Autodesk Inventor part; units mm, degrees
ref_plane "YZ Plane" through (0, 0, 0) normal (1, 0, 0) x (0, 1, 0)
ref_plane "XZ Plane" through (0, 0, 0) normal (0, 1, 0) x (-1, 0, 0)
ref_plane "XY Plane" through (0, 0, 0) normal (0, 0, 1) x (1, 0, 0)
sketch "Sketch1" plane through (0, 0, 0) normal (0, 1, 0) x (-1, 0, 0)
  line L0 (0, 0) -> (29.6, 0)
  line L1 (29.6, 0) -> (29.6, 24.2)
  line L2 (29.6, 24.2) -> (0, 24.2)
  line L3 (0, 24.2) -> (0, 0)
  line L4 (29.6, 12.5) -> (0, 12.5)
  line L5 (0, 12.5) -> (0, 0)
  line L6 (0, 0) -> (29.6, 0)
  line L7 (29.6, 0) -> (29.6, 12.5)
  line L8 (23.8, 24.2) -> (10.8, 24.2)
  line L9 (10.8, 24.2) -> (10.8, 12.5)
  line L10 (10.8, 12.5) -> (23.8, 12.5)
  line L11 (23.8, 12.5) -> (23.8, 24.2)
  line L12 (23.8, 17.7) -> (17.8, 17.7)
  line L13 (17.8, 17.7) -> (17.8, 12.5)
  line L14 (17.8, 12.5) -> (23.8, 12.5)
  line L15 (23.8, 12.5) -> (23.8, 17.7)
  line L16 (17.8, 17.7) -> (10.8, 17.7)
  line L17 (10.8, 17.7) -> (10.8, 12.5)
  line L18 (10.8, 12.5) -> (17.8, 12.5)
  line L19 (17.8, 12.5) -> (17.8, 17.7)
  circle A0 centre (21.6, 8) radius 8
  circle A1 centre (5, 7.5) radius 5
  circle A2 centre (16.3, 14) radius 1.5
  circle A3 centre (16.3, 16.2) radius 1.5
  circle A4 centre (26.8, 15.5) radius 3
  circle A5 centre (22.3, 22.7) radius 1.5
  circle A6 centre (11.8, 18.7) radius 1
  line L20 (10.8, 24.2) -> (15.8, 24.2)
  line L21 (15.8, 24.2) -> (15.8, 20.95)
  line L22 (15.8, 20.95) -> (10.8, 20.95)
  line L23 (10.8, 20.95) -> (10.8, 24.2)
  arc A7 (15.8, 24.2) -> (10.8, 20.95) centre (17.6697, 15.8525) ccw
  circle A8 centre (28.1, 11) radius 1.5
  point P0 (17.8, 14)
  point P1 (16.3, 12.5)
  point P2 (5, 12.5)
  point P3 (0, 7.5)
  point P4 (21.6, 0)
  point P5 (29.6, 8)
  point P6 (26.8, 12.5)
  point P7 (23.8, 15.5)
  point P8 (23.8, 22.7)
  point P9 (22.3, 24.2)
  point P10 (10.8, 18.7)
  point P11 (11.8, 17.7)
  point P12 (16.3, 17.7)
  point P13 (17.8, 16.2)
  point P14 (29.6, 11)
  point P15 (28.1, 12.5)
  dimension "d0" = 24.2
  dimension "d1" = 29.6
  dimension "d2" = 11.7
  dimension "d3" = 5.8
  dimension "d4" = 13
  dimension "d5" = 6.5
  dimension "d6" = 6
  dimension "d7" = 16
  dimension "d8" = 8
  dimension "d9" = 8
  dimension "d10" = 10
  dimension "d11" = 5
  dimension "d12" = 5
  dimension "d13" = 3
  dimension "d14" = 3
  dimension "d15" = 1.5
  dimension "d16" = 1.5
  dimension "d17" = 1.5
  dimension "d18" = 1.5
  dimension "d19" = 6
  dimension "d20" = 3
  dimension "d21" = 3
  dimension "d23" = 1.5
  dimension "d24" = 1.5
  dimension "d25" = 2
  dimension "d26" = 1
  dimension "d27" = 1
  dimension "d28" = 5
  dimension "d29" = 3.25
  dimension "d32" = 3
  dimension "d33" = 1.5
  dimension "d34" = 1.5
  dimension "d35" = 12.5
  dimension "d36" = 3
extrude "Extrusion1" add sketch "Sketch1" along normal blind 3 contours L3 A1 L4 A0 L0 | A0 L4 A8 | A1 | A0 A8 L1 | A2 L13 L4 | A8 A0 | A8 A0 | L13 A0 L11 L4 | L11 A4 L4 | L13 L12 L11 A0 | L9 L22 L21 L2 A5 L11 L12 L16 A6 | A6 | L16 L13 A3 | L21 L22 A7 | A5 picked at (19.8309, 8.6369)
properties part number "Pi_mount_newupper"
Could you check a few things on this model? Use its own coordinates, in mm. A direction names the side the tool comes from. Round coordinates to 2 decimals unless told otherwise and drop trailing zeros. Write each loop counter-clockwise with the first axis right and the second up, starting at its lowest first coordinate (ties: lowest second). Pieces come first, ordered by that corner, then holes. Notation, with made-up numbers: (-6, 26.25) - (3, 26.25) arc R4 cw to (3, 30.25) - close; hole circle Ø10 at (62, 79). An arc over 180 degrees is marked (long way). Put each result on its own line as item: value. Start each with the question number.
(1) For faces 1 (the flat face through (-10.8, 1, 20)), 2 (the cylindrical face through (-27.319, 1.479, 2.406)), 3 (the flat face through (-27, 1, 12.5)), 4 (the cylindrical face through (-17.35, 1.48, 17.27)), which set-ups out of +Z, -Z, +X, -X, +Y, -Y let a thin tool reach every point of the face, with its end or its side?
(2) I want a section at A-A, the plane x = -11.25. Please give me the cut outline in (y, z).
(3) Thinking about a two-plate mould opening in Z: for faces 5 (the flat face through (-15, 0, 10)), 6 (the flat face through (-17.8, 1, 15)), 7 (the flat face through (-11, 1, 0)), which applies, released by +Z, released by -Z, zero draft, split by the parting line, or undercut?
(4) I want a section at C-C, the plane z = 10.5. Please give me the cut outline in (x, y).
(5) Will these pins go through, and if not, where does the flat tip stop? pin 1 (1.1 mm diameter, centred on y = 1.5, z = 14.5, fed in from +X); pin 2 (5 mm diameter, centred on x = -10, z = 12.5, fed in from -Y); pin 3 (1 mm diameter, centred on x = -27, y = 2, fed in from +Z); pin 4 (1.5 mm diameter, centred on y = 0.5, z = 5.5, fed in from -X).
(6) I need wall thicknesses on probe 1 along Z at (x, y) = (-9.25, 2.2); probe 2 along X at (y, z) = (2, 15.5); probe 3 along X at (y, z) = (1.6, 18.75). Which ranges of each line are inside material? Lowest first, please.
(7) I want a section at B-B, the plane y = 0.5. Please give me the cut outline in (x, z), plus the area to 3 significant figures.
(8) I want a section at D-D, the plane z = 17. Please give me the cut outline in (x, y).
Here are the results:
1. face 1: +Z, +X, +Y, -Y
1. face 2: -Z, -X, +Y, -Y
1. face 3: +Z, -X, +Y, -Y
1. face 4: +X, +Y, -Y
2. outline: (0, 0) - (3, 0) - (3, 12.5) - (0, 12.5) - close; (0, 17.86) - (3, 17.86) - (3, 21.51) - (0, 21.51) - close
3. face 5: zero draft
3. face 6: undercut
3. face 7: released by -Z
4. outline: (-29.6, 0) - (-1, 0) - (-1, 3) - (-29.6, 3) - close
5. pin 1: stops at x = -17.8
5. pin 2: stops at y = 0
5. pin 3: stops at z = 12.52
5. pin 4: stops at x = -29.41
6. probe 1: z = 0 to 12.5
6. probe 2: x = -23.8 to -17.8
6. probe 3: x = -23.8 to -10.8
7. outline: (-29.6, 8) arc R8 ccw to (-21.6, 0) - (0, 0) - (0, 7.5) arc R5 ccw to (-5, 12.5) - (-16.3, 12.5) arc R1.5 cw to (-17.8, 14) - (-17.8, 16.2) arc R1.5 cw to (-16.3, 17.7) - (-11.8, 17.7) arc R1 ccw to (-10.8, 18.7) - (-10.8, 20.95) arc R8.55 ccw to (-15.8, 24.2) - (-22.3, 24.2) arc R1.5 ccw to (-23.8, 22.7) - (-23.8, 15.5) arc R3 cw to (-26.8, 12.5) - (-28.1, 12.5) arc R1.5 ccw to (-29.6, 11) - close
7. area: 462 mm^2
8. outline: (-23.8, 0) - (-17.57, 0) - (-17.57, 3) - (-23.8, 3) - close
